```python
from build123d import *

# Parameters (mm, degrees)
SKETCH_1_W          = 36
SKETCH_1_H          = 9.8
EXTRUDE_1_DEPTH     = 30
SKETCH_2_W          = 2.5
SKETCH_2_H          = 26
CUT_EXTRUDE_1_DEPTH = 48.116982077
SKETCH_3_W          = 24
SKETCH_3_H          = 26
CUT_EXTRUDE_2_DEPTH = 37.332354727
CUT_EXTRUDE_3_DEPTH = 3
CUT_EXTRUDE_4_REACH = 34.818
SKETCH_9_R          = 1


with BuildPart() as part:
    # 草图1 → 凸台-拉伸1 (new body)
    with BuildSketch(Plane(origin=(0, 0, 0), x_dir=(1, 0, 0), z_dir=(0, 1, 0))):
        Rectangle(SKETCH_1_W, SKETCH_1_H)
    extrude(amount=EXTRUDE_1_DEPTH)

    # 草图2 → 切除-拉伸1 (cut, through all)
    with BuildSketch(Plane(origin=(18, 0, 0), x_dir=(0, 0, -1), z_dir=(1, 0, 0))):
        with Locations((0, 17)):
            Rectangle(SKETCH_2_W, SKETCH_2_H)
    extrude(amount=-CUT_EXTRUDE_1_DEPTH, mode=Mode.SUBTRACT)

    # 草图3 → 切除-拉伸2 (cut, through all)
    with BuildSketch(Plane(origin=(0, 0, -4.9), x_dir=(-1, 0, 0), z_dir=(0, 0, -1))):
        with Locations((0, 17)):
            Rectangle(SKETCH_3_W, SKETCH_3_H)
    extrude(amount=-CUT_EXTRUDE_2_DEPTH, mode=Mode.SUBTRACT)

    # 草图5 → 切除-拉伸3 (cut)
    with BuildSketch(Plane.XZ):
        with BuildLine():
            Line((14.966101695, 2.113983221), (0.368644068, 3.606206671))
            ThreePointArc((0.368644068, 3.606206671), (0, 3.625), (-0.368644068, 3.606206671))
            Line((-0.368644068, 3.606206671), (-14.966101695, 2.113983221))
            ThreePointArc((-14.966101695, 2.113983221), (-16.875, 0), (-14.966101695, -2.113983221))
            Line((-14.966101695, -2.113983221), (-0.368644068, -3.606206671))
            ThreePointArc((-0.368644068, -3.606206671), (0, -3.625), (0.368644068, -3.606206671))
            Line((0.368644068, -3.606206671), (14.966101695, -2.113983221))
            ThreePointArc((14.966101695, -2.113983221), (16.875, 0), (14.966101695, 2.113983221))
        make_face()
    extrude(amount=-CUT_EXTRUDE_3_DEPTH, mode=Mode.SUBTRACT)

    # 草图9 → 切除-拉伸4 (cut, up to next)
    with BuildSketch(Plane.XZ.offset(-3), mode=Mode.PRIVATE) as cut_extrude_4_sk1:
        with Locations(Location((12.6, 0, 0), (0, 0, 270))):
            Circle(SKETCH_9_R)
    cut_extrude_4_tool1 = extrude(cut_extrude_4_sk1.sketch, amount=-CUT_EXTRUDE_4_REACH, mode=Mode.PRIVATE) & part.part
    # 草图9 → 切除-拉伸4 (cut, up to next)
    with BuildSketch(Plane.XZ.offset(-3), mode=Mode.PRIVATE) as cut_extrude_4_sk2:
        with Locations(Location((-12.6, 0, 0), (0, 0, 270))):
            Circle(SKETCH_9_R)
    cut_extrude_4_tool2 = extrude(cut_extrude_4_sk2.sketch, amount=-CUT_EXTRUDE_4_REACH, mode=Mode.PRIVATE) & part.part
    add(cut_extrude_4_tool1.solids().sort_by_distance((12.6, 3, 0))[0], mode=Mode.SUBTRACT)
    add(cut_extrude_4_tool2.solids().sort_by_distance((-12.6, 3, 0))[0], mode=Mode.SUBTRACT)


solid = part.part
```
Build history of the part. All positions in model axes, mm. A direction names the side the tool comes from. Coordinates: 2 decimals unless noted, no trailing zeros. Write each loop counter-clockwise with the first axis right and the second up, starting at its lowest first coordinate (ties: lowest second). Pieces come first, ordered by that corner, then holes.
1. Band-saw the part on A-A, the plane z = 0. Give the cut face in (x, y) (3 decimals), and give its area (4 significant figures).
Answer block:
outline: (-18, 0) - (-16.875, 0) - (-16.875, 3) - (-13.6, 3) - (-13.6, 4) - (-18, 4) - close; (-11.6, 3) - (11.6, 3) - (11.6, 4) - (-11.6, 4) - close; (13.6, 3) - (16.875, 3) - (16.875, 0) - (18, 0) - (18, 4) - (13.6, 4) - close
area: 38.75 mm2
2. Drop flat-ended pins along their axis: pin 1 (3 mm diameter, centred on x = 7, z = -2, fed in from +Y); pin 2 (3 mm diameter, centred on x = -11, z = -1, fed in from +Y). Give the stop position or say it passes through.
Answer block:
pin 1: stops at y = 4
pin 2: stops at y = 30
3. Pull direction Z, two halves, no side cores. Call faces 6 (the flat face through (-7.77, 1.48, -2.85)), 7 (the flat face through (-15, 30, -3)), 8 (the flat face through (0, 3, 0)), 9 (the flat face through (-12.3, 11.5, -4.9)): released by +Z, released by -Z, zero draft, split by the parting line, or undercut.
Answer block:
face 6: undercut
face 7: zero draft
face 8: undercut
face 9: released by -Z
4. Band-saw the part on C-C, the plane x = 12.6. Give the cut face in (y, z), and give its area (3 significant figures).
Answer block:
outline: (0, -4.9) - (30, -4.9) - (30, -1.25) - (4, -1.25) - (4, -1) - (3, -1) - (3, -2.36) - (0, -2.36) - close; (0, 2.36) - (3, 2.36) - (3, 1) - (4, 1) - (4, 1.25) - (30, 1.25) - (30, 4.9) - (0, 4.9) - close
area: 213 mm2
5. Band-saw the part on D-D, the plane x = -5. Give the cut face in (y, z), and give its area (3 significant figures).
Answer block:
outline: (0, -4.9) - (4, -4.9) - (4, 4.9) - (0, 4.9) - (0, 3.13) - (3, 3.13) - (3, -3.13) - (0, -3.13) - close
area: 20.4 mm2
6. 3-axis set-ups, long thin cutter, end or side, ignore diameter. For faces 1 (the flat face through (15, 17, -1.25)), 2 (the flat face through (15, 30, 3)), 3 (the cylindrical face through (16.875, 1.479, -0.044)), 4 (the flat face through (-12.3, 11.5, 4.9)), 5 (the flat face through (-12, 17, -3)): which of +Z, -Z, +X, -X, +Y, -Y reach the whole face in a straight line?
Answer block:
face 1: +X, -X, +Y
face 2: +Z, -Z, +X, -X, +Y
face 3: -Y
face 4: +Z, +X, -X, +Y, -Y
face 5: +Z, -Z, +Y
7. Drill centre lines: probe 1 along X at (y, z) = (3.35, 0); probe 2 along Z at (x, y) = (-15.5, 22.25); probe 3 along X at (y, z) = (24, -1.5). Where is each one in solid material? Low to high.
Answer block:
probe 1: x = -18 to -13.6, -11.6 to 11.6, 13.6 to 18
probe 2: z = -4.9 to -1.25, 1.25 to 4.9
probe 3: x = -18 to -12, 12 to 18
8. Band-saw the part on B-B, the plane y = 19.5. Give the cut face in (x, z).
Answer block:
outline: (-18, -4.9) - (-12, -4.9) - (-12, -1.25) - (-18, -1.25) - close; (-18, 1.25) - (-12, 1.25) - (-12, 4.9) - (-18, 4.9) - close; (12, -4.9) - (18, -4.9) - (18, -1.25) - (12, -1.25) - close; (12, 1.25) - (18, 1.25) - (18, 4.9) - (12, 4.9) - close
